The model under review builds one solid part; all positions refer to its coordinate system, in mm. A direction names the side the tool comes from. Round coordinates to 2 decimals unless told otherwise and drop trailing zeros. Order: outer loops, then holes, each group sorted by start corner. A loop starts at its lowest first (then second) coordinate and runs counter-clockwise, first axis right, second up.
Autodesk Inventor part; units mm, degrees
ref_plane "YZ Plane" through (0, 0, 0) normal (1, 0, 0) x (0, 1, 0)
ref_plane "XZ Plane" through (0, 0, 0) normal (0, 1, 0) x (-1, 0, 0)
ref_plane "XY Plane" through (0, 0, 0) normal (0, 0, 1) x (1, 0, 0)
sketch "Sketch1" plane through (0, 0, 0) normal (0, 1, 0) x (-1, 0, 0)
  circle A0 centre (0, 0) radius 4.5
  circle A1 centre (0, 0) radius 11
  circle A2 centre (0, 0) radius 6
  circle A3 centre (0, 0) radius 10.5
  line L0 (0, 0) -> (11, 0) construction
  line L1 (5.9161, 1) -> (10.9545, 1)
  line L2 (10.9545, 1) -> (10.9545, -1) construction
  line L3 (10.9545, -1) -> (5.9161, -1)
  line L4 (5.9161, -1) -> (5.9161, 1) construction
  line L5 (5.9161, 1) -> (10.9545, -1) construction
  line L6 (10.9545, 1) -> (5.9161, -1) construction
  line L7 (9.9868, 4.6112) -> (5.6235, 2.092)
  line L8 (4.6235, 3.8241) -> (8.9868, 6.3433)
  line L9 (6.3433, 8.9868) -> (3.8241, 4.6235)
  line L10 (2.092, 5.6235) -> (4.6112, 9.9868)
  line L11 (1, 10.9545) -> (1, 5.9161)
  line L12 (-1, 5.9161) -> (-1, 10.9545)
  line L13 (-4.6112, 9.9868) -> (-2.092, 5.6235)
  line L14 (-3.8241, 4.6235) -> (-6.3433, 8.9868)
  line L15 (-8.9868, 6.3433) -> (-4.6235, 3.8241)
  line L16 (-5.6235, 2.092) -> (-9.9868, 4.6112)
  line L17 (-10.9545, 1) -> (-5.9161, 1)
  line L18 (-5.9161, -1) -> (-10.9545, -1)
  line L19 (-9.9868, -4.6112) -> (-5.6235, -2.092)
  line L20 (-4.6235, -3.8241) -> (-8.9868, -6.3433)
  line L21 (-6.3433, -8.9868) -> (-3.8241, -4.6235)
  line L22 (-2.092, -5.6235) -> (-4.6112, -9.9868)
  line L23 (-1, -10.9545) -> (-1, -5.9161)
  line L24 (1, -5.9161) -> (1, -10.9545)
  line L25 (4.6112, -9.9868) -> (2.092, -5.6235)
  line L26 (3.8241, -4.6235) -> (6.3433, -8.9868)
  line L27 (8.9868, -6.3433) -> (4.6235, -3.8241)
  line L28 (5.6235, -2.092) -> (9.9868, -4.6112)
  line L29 (10.2705, -2.1831) -> (10.7596, -2.287)
  line L30 (10.2705, 2.1831) -> (10.7596, 2.287)
  line L31 (9.9861, 3.2447) -> (10.4616, 3.3992)
  line L32 (7.803, 7.0259) -> (8.1746, 7.3604)
  line L33 (7.0259, 7.803) -> (7.3604, 8.1746)
  line L34 (3.2447, 9.9861) -> (3.3992, 10.4616)
  line L35 (2.1831, 10.2705) -> (2.287, 10.7596)
  line L36 (-2.1831, 10.2705) -> (-2.287, 10.7596)
  line L37 (-3.2447, 9.9861) -> (-3.3992, 10.4616)
  line L38 (-7.0259, 7.803) -> (-7.3604, 8.1746)
  line L39 (-7.803, 7.0259) -> (-8.1746, 7.3604)
  line L40 (-9.9861, 3.2447) -> (-10.4616, 3.3992)
  line L41 (-10.2705, 2.1831) -> (-10.7596, 2.287)
  line L42 (-10.2705, -2.1831) -> (-10.7596, -2.287)
  line L43 (-9.9861, -3.2447) -> (-10.4616, -3.3992)
  line L44 (-7.803, -7.0259) -> (-8.1746, -7.3604)
  line L45 (-7.0259, -7.803) -> (-7.3604, -8.1746)
  line L46 (-3.2447, -9.9861) -> (-3.3992, -10.4616)
  line L47 (-2.1831, -10.2705) -> (-2.287, -10.7596)
  line L48 (2.1831, -10.2705) -> (2.287, -10.7596)
  line L49 (3.2447, -9.9861) -> (3.3992, -10.4616)
  line L50 (7.0259, -7.803) -> (7.3604, -8.1746)
  line L51 (7.803, -7.0259) -> (8.1746, -7.3604)
  line L52 (9.9861, -3.2447) -> (10.4616, -3.3992)
  point P0 (8.4353, 0)
  point P1 (8.4353, 1)
  point P2 (6.8052, 5.0837)
  point P3 (3.3516, 7.8052)
  point P4 (-1, 8.4353)
  point P5 (-5.0837, 6.8052)
  point P6 (-7.8052, 3.3516)
  point P7 (-8.4353, -1)
  point P8 (-6.8052, -5.0837)
  point P9 (-3.3516, -7.8052)
  point P10 (1, -8.4353)
  point P11 (5.0837, -6.8052)
  point P12 (7.8052, -3.3516)
  point P13 (9.9861, -3.2447)
  point P14 (9.5519, -4.3601)
  point P15 (10.4523, -1)
  point P16 (10.2705, 2.1831)
  point P17 (10.4523, 1)
  point P18 (9.5519, 4.3601)
  point P19 (9.9861, 3.2447)
  point P20 (7.803, 7.0259)
  point P21 (8.5519, 6.0922)
  point P22 (6.0922, 8.5519)
  point P23 (7.0259, 7.803)
  point P24 (3.2447, 9.9861)
  point P25 (4.3601, 9.5519)
  point P26 (1, 10.4523)
  point P27 (2.1831, 10.2705)
  point P28 (-1, 10.4523)
  point P29 (-4.3601, 9.5519)
  point P30 (-6.0922, 8.5519)
  point P31 (-8.5519, 6.0922)
  point P32 (-7.803, 7.0259)
  point P33 (-9.9861, 3.2447)
  point P34 (-9.5519, 4.3601)
  point P35 (-10.4523, 1)
  point P36 (-10.2705, 2.1831)
  point P37 (-10.2705, -2.1831)
  point P38 (-10.4523, -1)
  point P39 (-9.5519, -4.3601)
  point P40 (-9.9861, -3.2447)
  point P41 (-7.803, -7.0259)
  point P42 (-8.5519, -6.0922)
  point P43 (-6.0922, -8.5519)
  point P44 (-7.0259, -7.803)
  point P45 (-3.2447, -9.9861)
  point P46 (-4.3601, -9.5519)
  point P47 (-1, -10.4523)
  point P48 (-2.1831, -10.2705)
  point P49 (2.1831, -10.2705)
  point P50 (1, -10.4523)
  point P51 (4.3601, -9.5519)
  point P52 (3.2447, -9.9861)
  point P53 (6.0922, -8.5519)
  point P54 (8.5519, -6.0922)
  point P55 (7.803, -7.0259)
  dimension "d1" = 22
  dimension "d2" = 12
  dimension "d3" = 0.5
  dimension "d0" = 9
  dimension "d4" = 2
  dimension "d7" = 360
  dimension "d9" = 12
  dimension "d12" = 360
extrude "Extrusion1" add sketch "Sketch1" along normal blind 5 contours A1 L3 A3 L1 | L1 A3 L30 A1 | A1 L29 A3 L3 | A3 L3 A2 L1 | L31 A3 L7 A1 | A2 | A1 L28 A3 L52 | L7 A3 L8 A1 | A2 L8 A3 L7 | A1 L27 A3 L28 | L28 A3 L27 A2 | L8 A3 L32 A1 | A1 L51 A3 L27 | A2 L10 A3 L9 | L26 A3 L25 A2 | L33 A3 L9 A1 | A3 L10 A1 L9 | A1 L26 A3 L50 | L26 A1 L25 A3 | A2 L12 A3 L11 | A3 L34 A1 L10 | L24 A3 L23 A2 | L25 A1 L49 A3 | L11 A1 L35 A3 | A3 L12 A1 L11 | L24 A1 L23 A3 | A3 L48 A1 L24 | A2 L14 A3 L13 | A3 L36 A1 L12 | L22 A3 L21 A2 | L23 A1 L47 A3 | L13 A1 L37 A3 | A3 L14 A1 L13 | L22 A1 L21 A3 | A3 L46 A1 L22 | A2 L16 A3 L15 | A3 L38 A1 L14 | L20 A3 L19 A2 | L21 A1 L45 A3 | L15 A1 L39 A3 | A3 L16 A1 L15 | L20 A1 L19 A3 | A3 L44 A1 L20 | A2 L18 A3 L17 | A3 L40 A1 L16 | L19 A1 L43 A3 | L17 A1 L41 A3 | A3 L18 A1 L17 | A3 L42 A1 L18
sketch "Sketch2" plane through (0, 5, 0) normal (0, 1, 0) x (1, 0, 0)
  circle A0 centre (0, 0) radius 4.5
  circle A1 centre (0, 4.5) radius 0.5
  line L0 (0, 0) -> (0, 4.5) construction
  dimension "d16" = 1
extrude "Extrusion2" cut sketch "Sketch2" against normal through all contours A1 A0 | A0 A1 picked at (0.0194, 4.3324) picked at (0.0158, 4.6639)
properties part number "STATOR" material "Stainless Steel"
(1) Insertion check: pin 1 (3 mm diameter, centred on x = -3.5, y = 2.5, fed in from -Z); pin 2 (2 mm diameter, centred on x = -7.5, y = 3, fed in from -Z); pin 3 (2 mm diameter, centred on y = 3.5, z = -1.5, fed in from +X). Each pin has a flat end and moves straight along its axis. Give the tip position at first contact, or say it passes through.
Data:
pin 1: stops at z = -10.82
pin 2: stops at z = -8.87
pin 3: stops at x = 10.99
(2) Consider section A-A (z = 0). Write out the cut boundary in (x, y).
Data:
outline: (-11, 0) - (-4.5, 0) - (-4.5, 5) - (-11, 5) - close; (4.5, 0) - (11, 0) - (11, 5) - (4.5, 5) - close
(3) Consider section C-C (x = 9). Write out the cut boundary in (y, z).
Data:
outline: (0, -6.32) - (5, -6.32) - (5, -4.04) - (0, -4.04) - close; (0, -1) - (5, -1) - (5, 1) - (0, 1) - close; (0, 4.04) - (5, 4.04) - (5, 6.32) - (0, 6.32) - close
(4) To check wall thickness, follow probe 1 along X at (y, z) = (1.85, 0); probe 2 along Z at (x, y) = (0, 2.05); probe 3 along X at (y, z) = (4.15, -9). State the ranges of each line that lie inside material, in increasing order.
Data:
probe 1: x = -11 to -4.5, 4.5 to 11
probe 2: z = -11 to -5, 4.5 to 11
probe 3: x = -6.32 to -4.04, -1 to 1, 4.04 to 6.32
(5) Draft analysis for pull direction Z (two halves, no side actions). For faces 3 (the flat face through (-5, 5, 0)), 4 (the cylindrical face through (-10.377, 2.465, 1.602)), 5 (the cylindrical face through (-5.472, 2.465, 9.542)), state which applies: pulls with the +Z half, pulls with the -Z half, needs draft (parallel to the pull), parting line crosses it, or undercut.
Data:
face 3: needs draft
face 4: undercut
face 5: pulls with the +Z half
(6) For faces 1 (the cylindrical face through (5.53, 2.46, 9.51)), 2 (the cylindrical face through (10.377, 2.465, -1.602)), list the 3-axis set-ups (+Z, -Z, +X, -X, +Y, -Y) from which the entire face can be reached by the end or side of a thin tool; tool diameter is ignored.
Data:
face 1: +Z, +X, +Y, -Y
face 2: +Y, -Y
(7) Consider section B-B (x = 0). Write out the cut boundary in (y, z), and give its area (3 significant figures).
Data:
outline: (0, -11) - (5, -11) - (5, -5) - (0, -5) - close; (0, 4.5) - (5, 4.5) - (5, 11) - (0, 11) - close
area: 62.5 mm2
